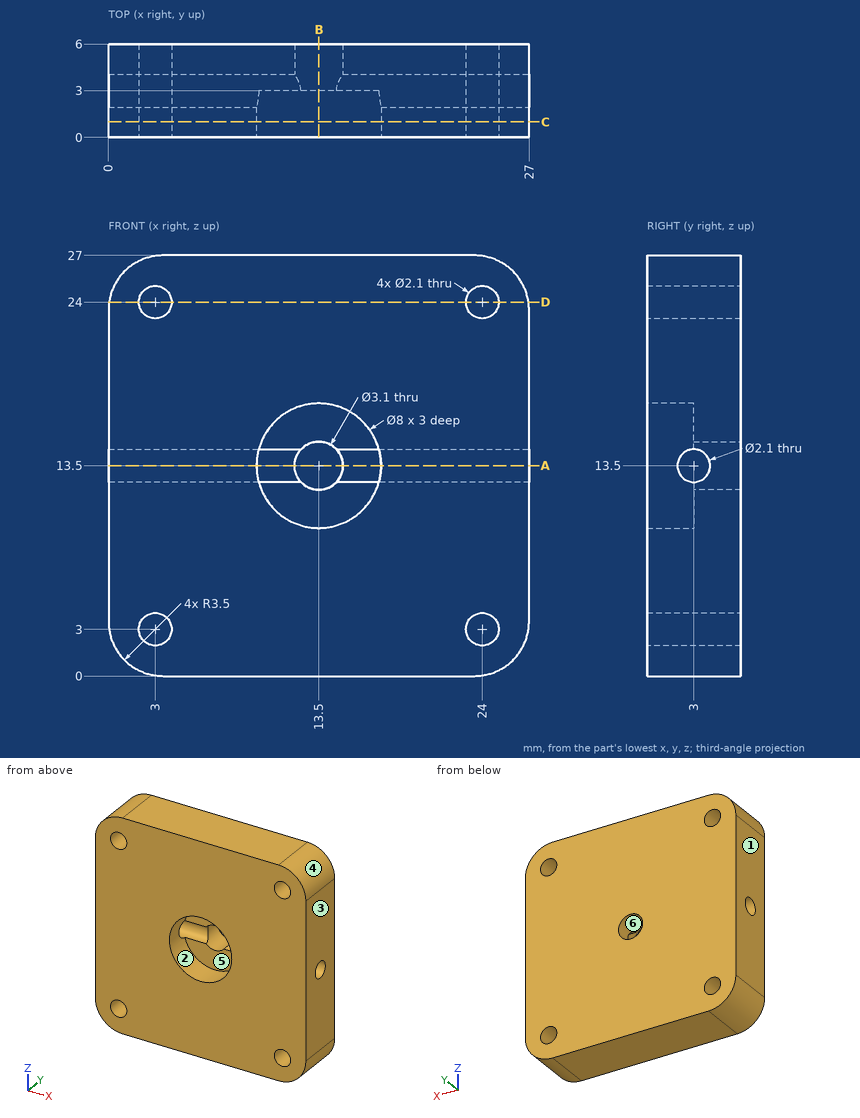
Can you work these out from the drawing? Everything is in mm from the part's minimum corner. A direction names the side the tool comes from. Give positions to 0.01 mm unless a question says otherwise; leave off trailing zeros. Loops run counter-clockwise (first coordinate to the right, second up) from the corner with the lowest first, then second, coordinate; pieces in that order, holes last. Notation, with made-up numbers: M 6.5,-4.75 L 62.5,-4.75 A27 cw 62.5,13.25 Z; hole C 45,42.25 d11. An arc over 180 degrees is marked long. Use CSV: the item, a comma, the result in double quotes. Start each with the question number.
1. On a 3-axis mill with a long thin cutter (end or side, diameter ignored), from which of +Z, -Z, +X, -X, +Y, -Y can I reach the whole of each face in a straight line? I mean the marked faces 1 and 2. Say none if no direction works.
2. Imagine slicing it at D-D, the plane z = 24. Write out the boundary of the cut face in (x, y).
3. Imagine slicing it at A-A, the plane z = 13.5. Write out the boundary of the cut face in (x, y), plus the area to 3 significant figures.
4. If we mould it in two halves opening along Z, with no side actions, what happens to the marked faces 3, 4, 5 and 6? For each: released by +Z, released by -Z, zero draft, split by the parting line, or undercut.
5. Imagine slicing it at C-C, the plane y = 1. Write out the boundary of the cut face in (x, z).
6. If I drill on L1, parallel to X at y = 1.55, z = 24; L2, parallel to Y at x = 8, z = 13.5; L3, parallel to Z at x = 3.75, y = 3.25, over which ranges is the centre line in solid material (lowest first)?
7. Imagine slicing it at B-B, the plane x = 13.5. Write out the boundary of the cut face in (y, z), plus the area to 3 significant figures.
8. For P1, Ø1.3, axis at y = 3, z = 13.5, coming from the +X side; P2, Ø3, axis at x = 14, z = 15.5, coming from the -Y side, each with a flat end and sliding along its axis, tell me the tip position at first contact or that it passes through.
Response values:
1,face 1,"+Z, -Z, -X, +Y, -Y"
1,face 2,"-Y"
2,outline,"M 0.04,0 L 1.95,0 L 1.95,6 L 0.04,6 Z; M 4.05,0 L 22.95,0 L 22.95,6 L 4.05,6 Z; M 25.05,0 L 26.96,0 L 26.96,6 L 25.05,6 Z"
3,outline,"M 0,0 L 9.5,0 L 9.5,1.95 L 0,1.95 Z; M 0,4.05 L 11.95,4.05 L 11.95,6 L 0,6 Z; M 15.05,4.05 L 27,4.05 L 27,6 L 15.05,6 Z; M 17.5,0 L 27,0 L 27,1.95 L 17.5,1.95 Z"
3,area,"83.7 mm^2"
4,face 3,"zero draft"
4,face 4,"released by +Z"
4,face 5,"undercut"
4,face 6,"undercut"
5,outline,"M 0,3.5 A3.5 ccw 3.5,0 L 23.5,0 A3.5 ccw 27,3.5 L 27,23.5 A3.5 ccw 23.5,27 L 3.5,27 A3.5 ccw 0,23.5 Z; hole C 3,3 d2.1; hole C 3,24 d2.1; hole C 13.5,13.5 d8; hole C 24,3 d2.1; hole C 24,24 d2.1"
6,L1,"0.04 to 1.95, 4.05 to 22.95, 25.05 to 26.96"
6,L2,"0 to 1.95, 4.05 to 6"
6,L3,"0 to 2.27, 3.73 to 12.48, 14.52 to 23.27, 24.73 to 27"
7,outline,"M 0,0 L 6,0 L 6,11.95 L 3,11.95 L 3,9.5 L 0,9.5 Z; M 0,17.5 L 3,17.5 L 3,15.05 L 6,15.05 L 6,27 L 0,27 Z"
7,area,"129 mm^2"
8,P1,"through"
8,P2,"y = 3"
